from build123d import *

# Parameters (mm, degrees)
SKETCH1_R             = 4
BOSS_EXTRUDE1_DEPTH   = 5
BOSS_EXTRUDE2_DEPTH   = 5
SKETCH7_R             = 15
SKETCH7_R_2           = 4
BOSS_EXTRUDE3_DEPTH   = 5
FILLET1_R             = 10
IZIM1_R               = 16
KES_EKSTR_ZYON1_DEPTH = 5


with BuildPart() as part:
    # Sketch1 → Boss-Extrude1 (new body)
    with BuildSketch(Plane.XY):
        with BuildLine():
            Line((44.539250231, 30.397114607), (14.976761962, 0.834626339))
            ThreePointArc((14.976761962, 0.834626339), (-10.606601718, -10.606601718), (0.834626339, 14.976761962))
            Line((0.834626339, 14.976761962), (36.254978983, 50.397114607))
            Line((36.254978983, 50.397114607), (213.745021017, 50.397114607))
            Line((213.745021017, 50.397114607), (249.165373661, 14.976761962))
            ThreePointArc((249.165373661, 14.976761962), (260.606601718, -10.606601718), (235.023238038, 0.834626339))
            Line((235.023238038, 0.834626339), (205.460749769, 30.397114607))
            Line((205.460749769, 30.397114607), (44.539250231, 30.397114607))
        make_face()
        Circle(SKETCH1_R, mode=Mode.SUBTRACT)
        with Locations((250, 0)):
            Circle(SKETCH1_R, mode=Mode.SUBTRACT)
    extrude(amount=BOSS_EXTRUDE1_DEPTH)

    # Sketch6 → Boss-Extrude2 (add)
    with BuildSketch(Plane.XY.offset(5)):
        Polygon((243.862072803, 9.673461103), (210.638419299, 42.897114607), (39.361580701, 42.897114607), (6.137927197, 9.673461103), (9.673461103, 6.137927197), (41.432648513, 37.897114607), (208.567351487, 37.897114607), (240.326538897, 6.137927197), align=None)
    extrude(amount=BOSS_EXTRUDE2_DEPTH)

    # Sketch7 → Boss-Extrude3 (add)
    # profile 1 of 2: a face of its own
    with BuildSketch(Plane.XY.offset(5)):
        Circle(SKETCH7_R)
        Circle(SKETCH7_R_2, mode=Mode.SUBTRACT)
    # profile 2 of 2: a face of its own
    with BuildSketch(Plane.XY.offset(5)):
        with Locations((250, 0)):
            Circle(SKETCH7_R)
        with Locations((250, 0)):
            Circle(SKETCH7_R_2, mode=Mode.SUBTRACT)
    extrude(amount=BOSS_EXTRUDE3_DEPTH)

    # Fillet1
    fillet1_edges = [part.edges().sort_by_distance(p)[0] for p in [
        (8.690483379, 12.226017285, 7.5),
        (12.226017285, 8.690483379, 7.5),
        (241.309516621, 12.226017285, 7.5),
        (237.773982715, 8.690483379, 7.5),
    ]]
    fillet(fillet1_edges, radius=FILLET1_R)

    # Çizim1 → Kes-Ekstrüzyon1 (cut)
    with BuildSketch(Plane.XY.offset(10)):
        with Locations((250, 0)):
            Circle(IZIM1_R)
    extrude(amount=-KES_EKSTR_ZYON1_DEPTH, mode=Mode.SUBTRACT)


solid = part.part
Input: part model. Units: mm. Frame: model coordinates. A direction names the side the tool comes from. Give positions to 0.01 mm unless a question says otherwise; leave off trailing zeros. Order: outer loops, then holes, each group sorted by start corner. A loop starts at its lowest first (then second) coordinate and runs counter-clockwise, first axis right, second up. Notation, with made-up numbers: (85.25, 34) - (122.25, 34) arc R24 cw to (122.25, 60) - close; hole circle Ø5 at (55, 17). An arc over 180 degrees is marked (long way). Write each question's results on one line, items separated by ' | '.
Item 1: Material intervals for line 1 along Y through (x, z) = (250, 1); line 2 along Y through (x, z) = (127, 0.5); line 3 along Y through (x, z) = (1, 3.5), sorted ascending.
A:
line 1: y = -15 to -4, 4 to 15 | line 2: y = 30.4 to 50.4 | line 3: y = -14.97 to -3.87, 3.87 to 15.14
Item 2: Draft query along Y for faces 5 (the flat face through (126, 42.897, 7)), 6 (the cylindrical face through (-0.867, -3.905, 4.93)), 7 (the flat face through (85, 40, 10)), 8 (the flat face through (126, 30.397, 2)). Return one class per face: released by +Y, released by -Y, zero draft, split by the parting line, or undercut.
A:
face 5: released by +Y | face 6: undercut | face 7: zero draft | face 8: released by -Y
Item 3: Contact query for flat-ended pins moving along their axis: pin 1 Ø2.5 at (x, z) = (108.5, 7.5) entering from -Y; pin 2 Ø4 at (x, z) = (142.5, 8.5) entering from +Y; pin 3 Ø5 at (x, y) = (31, 22.5) entering from +Z; pin 4 Ø12 at (x, y) = (226.5, 28) entering from +Z. Output: stop coordinate, or through.
A:
pin 1: stops at y = 37.9 | pin 2: stops at y = 42.9 | pin 3: stops at z = 5 | pin 4: stops at z = 10
Item 4: Section D-D (y = 40.5). Return loops of the section in (x, z), and give its area (3 significant figures).
A:
outline: (26.36, 0) - (223.64, 0) - (223.64, 5) - (213.04, 5) - (213.04, 10) - (36.96, 10) - (36.96, 5) - (26.36, 5) - close | area: 1,870 mm^2
Item 5: Section A-A (z = 3). Return loops of the section in (x, y).
A:
outline: (0.83, 14.98) arc R15 ccw (long way) to (14.98, 0.83) - (44.54, 30.4) - (205.46, 30.4) - (235.02, 0.83) arc R15 ccw (long way) to (249.17, 14.98) - (213.75, 50.4) - (36.25, 50.4) - close; hole circle Ø8 at (0, 0); hole circle Ø8 at (250, 0)
Item 6: Access query for faces 1 (the cylindrical face through (234.884, 10.763, 7.465)), 2 (the flat face through (143, 35, 5)), 3 (the cylindrical face through (8.99, 14.47, 7.46)), 4 (the flat face through (223.729, 29.806, 7.465)). Directions: +Z, -Z, +X, -X, +Y, -Y. A direction counts if a zero-diameter tool reaches every point of the face in a straight line with its end or side. Return the directions, or none.
A:
face 1: +Z, -Y | face 2: +Z | face 3: +Z, +Y | face 4: +Z, +X, +Y
Item 7: Section C-C (x = 153.5). Return loops of the section in (y, z).
A:
outline: (30.4, 0) - (50.4, 0) - (50.4, 5) - (42.9, 5) - (42.9, 10) - (37.9, 10) - (37.9, 5) - (30.4, 5) - close
Item 8: Section B-B (y = 25.5). Return loops of the section in (x, z), and give its area (3 significant figures).
A:
outline: (11.36, 0) - (39.64, 0) - (39.64, 5) - (29.04, 5) - (29.04, 10) - (21.96, 10) - (21.96, 5) - (11.36, 5) - close; (210.36, 0) - (238.64, 0) - (238.64, 5) - (228.04, 5) - (228.04, 10) - (220.96, 10) - (220.96, 5) - (210.36, 5) - close | area: 354 mm^2
